Study the drawing (mm; zero at the part's minimum x, y, z) and answer. A direction names the side the tool comes from. Give positions to 0.01 mm unless a question says otherwise; leave off trailing zeros. Write each loop counter-clockwise with the first axis right and the second up, starting at its lowest first coordinate (ties: lowest second). Pieces come first, ordered by that corner, then holes. Notation, with made-up numbers: (52.5, -22) -> (73.5, -22) arc R33 ccw to (73.5, 14) -> close; hole circle Ø7 at (43, -24.75). An arc over 180 degrees is marked (long way). Put each result on its own line as item: value. Start each with the question number.
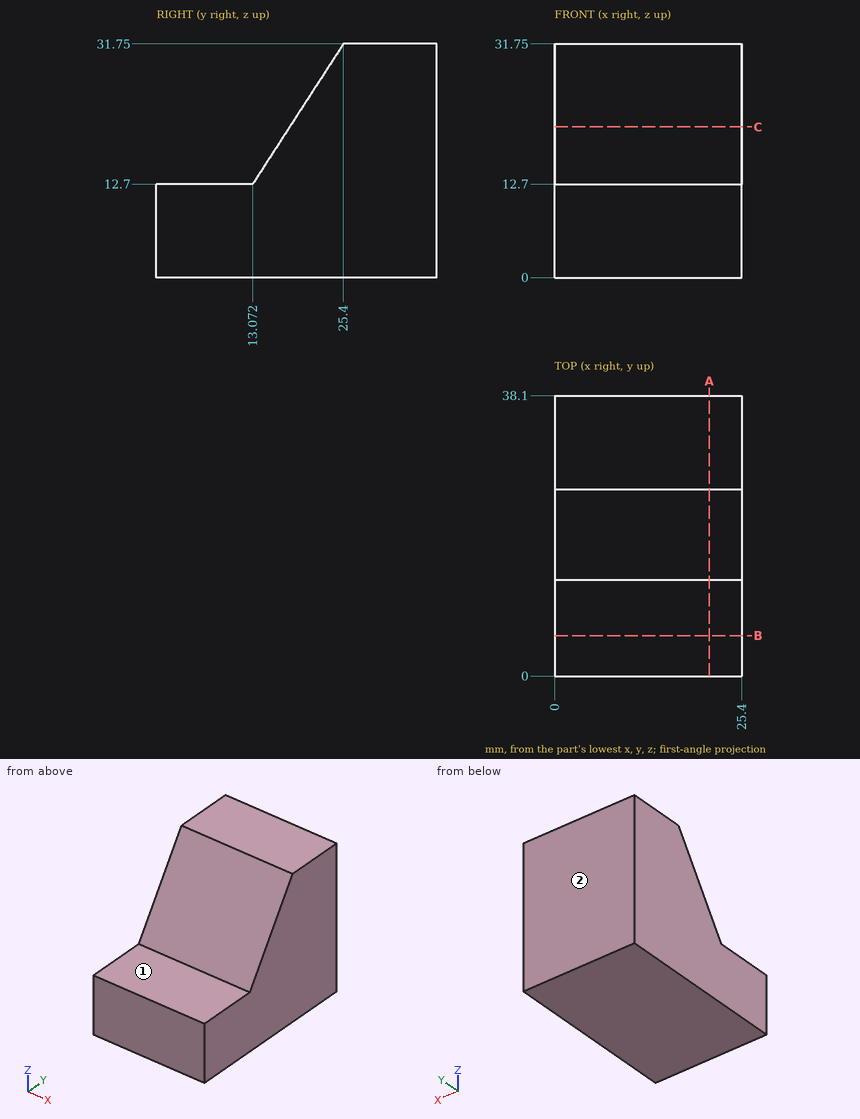
1) A cutting plane is placed at B-B on y = 5.5. Give the vertices of the cut face in (x, z), and give its area (3 significant figures).
2) Straight lines are drawn through the part: line 1 (Z direction, x = 18.5, y = 13); line 2 (Y direction, x = 22, z = 21.5); line 3 (Y direction, x = 8.75, z = 26.5). For each, find the intervals that lie inside material, in ascending order. Write a range as [from, to].
3) A cutting plane is placed at C-C on z = 20.5. Give the vertices of the cut face in (x, y).
4) Each of these flat-tipped pins is pushed along its axis until it touches: pin 1 Ø4 at (x, y) = (15, 5) entering from +Z; pin 2 Ø10 at (x, y) = (14, 16) entering from +Z. Where does it stop, or does it pass through?
5) For the marked faces 1 and 2, determine the directions among +Z, -Z, +X, -X, +Y, -Y from which every point of the face is accessible in a straight line to the end or side of a thin tool.
6) A cutting plane is placed at A-A on x = 21. Give the vertices of the cut face in (y, z), and give its area (3 significant figures).
Results found:
1. outline: (0, 0) -> (25.4, 0) -> (25.4, 12.7) -> (0, 12.7) -> close
1. area: 323 mm²
2. line 1: z = [0, 12.7]
2. line 2: y = [18.77, 38.1]
2. line 3: y = [22, 38.1]
3. outline: (0, 18.12) -> (25.4, 18.12) -> (25.4, 38.1) -> (0, 38.1) -> close
4. pin 1: stops at z = 12.7
4. pin 2: stops at z = 24.95
5. face 1: +Z, +X, -X, -Y
5. face 2: +Z, -Z, +X, -X, +Y
6. outline: (0, 0) -> (38.1, 0) -> (38.1, 31.75) -> (25.4, 31.75) -> (13.07, 12.7) -> (0, 12.7) -> close
6. area: 843 mm²
